Geometry: final body of the model. Coordinates: model frame, mm. A direction names the side the tool comes from. Coordinates: 2 decimals unless noted, no trailing zeros. Write each loop counter-clockwise with the first axis right and the second up, starting at its lowest first coordinate (ties: lowest second). Pieces come first, ordered by that corner, then holes.
Autodesk Inventor part; units mm, degrees
ref_plane "YZ Plane" through (0, 0, 0) normal (1, 0, 0) x (0, 1, 0)
ref_plane "XZ Plane" through (0, 0, 0) normal (0, 1, 0) x (-1, 0, 0)
ref_plane "XY Plane" through (0, 0, 0) normal (0, 0, 1) x (1, 0, 0)
sketch "Sketch1" plane through (0, 0, 0) normal (0, 0, 1) x (1, 0, 0)
  line L0 (-6.8404, -18.7939) -> (73.1596, -18.7939) construction
  line L1 (126.5636, -18.7939) -> (116.303, 9.3969)
  line L2 (27.3616, 75.1754) -> (20.5212, 56.3816)
  line L3 (20.5212, 56.3816) -> (24.28, 55.0135)
  line L4 (24.28, 55.0135) -> (20.8598, 45.6166)
  line L5 (20.8598, 45.6166) -> (17.101, 46.9846)
  line L6 (17.101, 46.9846) -> (10.2606, 28.1908)
  line L7 (10.2606, 28.1908) -> (14.0194, 26.8227)
  line L8 (14.0194, 26.8227) -> (10.5992, 17.4258)
  line L9 (10.5992, 17.4258) -> (6.8404, 18.7939)
  line L10 (6.8404, 18.7939) -> (-6.8404, -18.7939)
  line L11 (27.3616, 75.1754) -> (47.3616, 75.1754)
  line L12 (47.3616, 75.1754) -> (47.3616, 71.1754)
  line L13 (47.3616, 71.1754) -> (57.3616, 71.1754)
  line L14 (57.3616, 71.1754) -> (57.3616, 75.1754)
  line L15 (57.3616, 75.1754) -> (72.3616, 75.1754)
  line L16 (72.3616, 75.1754) -> (72.3616, 71.1754)
  line L17 (72.3616, 71.1754) -> (82.3616, 71.1754)
  line L18 (82.3616, 71.1754) -> (82.3616, 75.1754)
  line L19 (82.3616, 75.1754) -> (97.3616, 75.1754)
  line L20 (97.3616, 75.1754) -> (97.3616, 71.1754)
  line L21 (97.3616, 71.1754) -> (107.3616, 71.1754)
  line L22 (107.3616, 71.1754) -> (107.3616, 75.1754)
  line L23 (107.3616, 75.1754) -> (127.3616, 75.1754)
  line L24 (-6.8404, -18.7939) -> (3.1596, -18.7939)
  line L25 (3.1596, -18.7939) -> (3.1596, -14.7939)
  line L26 (3.1596, -14.7939) -> (18.1596, -14.7939)
  line L27 (18.1596, -14.7939) -> (18.1596, -18.7939)
  line L28 (28.1596, -18.7939) -> (18.1596, -18.7939)
  line L29 (38.4202, 9.3969) -> (35, 0)
  line L30 (35, 0) -> (31.2412, 1.3681)
  line L31 (31.2412, 1.3681) -> (27.821, -8.0288)
  line L32 (27.821, -8.0288) -> (31.5798, -9.3969)
  line L33 (31.5798, -9.3969) -> (28.1596, -18.7939)
  line L34 (38.4202, 9.3969) -> (50.5212, 9.3969)
  line L35 (50.5212, 9.3969) -> (50.5212, 13.3969)
  line L36 (50.5212, 13.3969) -> (60.5212, 13.3969)
  line L37 (60.5212, 13.3969) -> (60.5212, 9.3969)
  line L38 (116.303, 9.3969) -> (104.202, 9.3969)
  line L39 (104.202, 9.3969) -> (104.202, 13.3969)
  line L40 (104.202, 13.3969) -> (94.202, 13.3969)
  line L41 (94.202, 13.3969) -> (94.202, 9.3969)
  line L42 (60.5212, 9.3969) -> (94.202, 9.3969)
  line L43 (116.303, 9.3969) -> (119.7232, 0)
  line L44 (119.7232, 0) -> (123.482, 1.3681)
  line L45 (123.482, 1.3681) -> (126.9022, -8.0288)
  line L46 (126.9022, -8.0288) -> (123.1434, -9.3969)
  line L47 (123.1434, -9.3969) -> (126.5636, -18.7939)
  line L48 (126.5636, -18.7939) -> (136.5636, -18.7939)
  line L49 (136.5636, -18.7939) -> (136.5636, -14.7939)
  line L50 (136.5636, -14.7939) -> (151.5636, -14.7939)
  line L51 (151.5636, -14.7939) -> (151.5636, -18.7939)
  line L52 (161.5636, -18.7939) -> (151.5636, -18.7939)
  line L53 (127.3616, 75.1754) -> (134.202, 56.3816)
  line L54 (134.202, 56.3816) -> (130.4432, 55.0135)
  line L55 (130.4432, 55.0135) -> (133.8634, 45.6166)
  line L56 (133.8634, 45.6166) -> (137.6222, 46.9846)
  line L57 (137.6222, 46.9846) -> (144.4626, 28.1908)
  line L58 (144.4626, 28.1908) -> (140.7038, 26.8227)
  line L59 (140.7038, 26.8227) -> (144.124, 17.4258)
  line L60 (144.124, 17.4258) -> (147.8828, 18.7939)
  line L61 (147.8828, 18.7939) -> (161.5636, -18.7939)
  dimension "d22" = 100
  dimension "d24" = 100
  dimension "d27" = 35
  dimension "d28" = 30
  dimension "d29" = 35
  dimension "d30" = 30
  dimension "d32" = 20
  dimension "d33" = 4
  dimension "d34" = 10
  dimension "d35" = 20
  dimension "d36" = 10
  dimension "d37" = 20
  dimension "d38" = 4
  dimension "d39" = 10
  dimension "d40" = 15
  dimension "d41" = 10
  dimension "d42" = 15
  dimension "d43" = 10
  dimension "d49" = 10
  dimension "d50" = 4
  dimension "d51" = 15
  dimension "d52" = 10
  dimension "d53" = 4
  dimension "d54" = 10
  dimension "d55" = 12.101
  dimension "d56" = 4
  dimension "d57" = 10
  dimension "d58" = 12.101
  dimension "d59" = 10
  dimension "d60" = 10
  dimension "d62" = 10
  dimension "d63" = 10
  dimension "d64" = 4
  dimension "d65" = 15
  dimension "d68" = 20
  dimension "d69" = 4
  dimension "d70" = 10
  dimension "d71" = 20
  dimension "d72" = 4
  dimension "d73" = 10
extrude "Extrusion1" add sketch "Sketch1" along normal blind 4 contours L1 L46 L45 L44 L38 L39 L40 L41 L42 L37 L36 L35 L34 L29 L30 L31 L32 L33 L28 L27 L26 L25 L24 L10 L9 L8 L7 L6 L5 L4 L3 L2 L11 L12 L13 L14 L15 L16 L17 L18 L19 L20 L21 L22 L23 L53 L54 L55 L56 L57 L58 L59 L60 L61 L52 L51 L50 L49 L48
properties part number "back"
Item 1: Section A-A, the plane x = 112.5. Output: boundary loops of the cut face in (y, z), plus the area to 3 significant figures.
Derived:
outline: (9.4, 0) - (75.18, 0) - (75.18, 4) - (9.4, 4) - close
area: 263 mm2
Item 2: Section B-B, the plane y = 60. Output: boundary loops of the cut face in (x, z) (3 decimals), plus the area to 3 significant figures.
Derived:
outline: (21.838, 0) - (132.885, 0) - (132.885, 4) - (21.838, 4) - close
area: 444 mm2
Item 3: Material intervals for probe 1 along Y at (x, z) = (97.5, 1.6); probe 2 along Y at (x, z) = (46, 3.7); probe 3 along X at (y, z) = (66.5, 1.2), sorted ascending.
Derived:
probe 1: y = 13.4 to 71.18
probe 2: y = 9.4 to 75.18
probe 3: x = 24.2 to 130.52
Item 4: Set-up query: faces 4 (the flat face through (57.362, 73, 2)), 5 (the flat face through (125.049, -8.703, 1.972)), 6 (the flat face through (110, 9.397, 2)), 7 (the flat face through (65, 75.175, 2)). Return all of +Z, -Z, +X, -X, +Y, -Y with unobstructed straight access to the full face (end or side cutting, diameter ignored); none if empty.
Derived:
face 4: +Z, -Z, +Y
face 5: +Z, -Z
face 6: +Z, -Z, -Y
face 7: +Z, -Z, +X, -X, +Y
Item 5: Pull-direction query (X, two-part tool) for faces 1 (the flat face through (117, 75.175, 2)), 2 (the flat face through (19.01, 46.29, 1.97)), 3 (the flat face through (77, 71.175, 2)); classes: released by +X, released by -X, zero draft, split by the parting line, or undercut.
Derived:
face 1: zero draft
face 2: undercut
face 3: undercut
Item 6: Pin query (flat end, axial travel): pin 1 (2 mm diameter, centred on y = 11, z = 2, fed in from -X); pin 2 (2 mm diameter, centred on x = 57.5, z = 2.5, fed in from -Y); pin 3 (1.2 mm diameter, centred on y = -16, z = 3, fed in from -X); pin 4 (1.5 mm diameter, centred on x = 35, y = 60, fed in from -Z). Return the tip coordinate at first contact, or that it passes through.
Derived:
pin 1: stops at x = 3.64
pin 2: stops at y = 13.4
pin 3: stops at x = -6.04
pin 4: stops at z = 0
